```python
from build123d import *

# Parameters (mm, degrees)
BOSS_EXTRU_3_DEPTH      = 30
ESQUISSE2_W             = 15
ESQUISSE2_H             = 50
BOSS_EXTRU_4_DEPTH      = 30
CONG_1_R                = 5
ESQUISSE3_R             = 4
ENL_V_MAT_EXTRU_1_DEPTH = 30
ESQUISSE4_R             = 4
ENL_V_MAT_EXTRU_2_DEPTH = 30
CONG_2_R                = 0.5
ESQUISSE5_R             = 3
ENL_V_MAT_EXTRU_3_DEPTH = 30


with BuildPart() as part:
    # Esquisse1 → Boss.-Extru.3 (new body)
    with BuildSketch(Plane.XY):
        with BuildLine():
            Line((-1.516636282, -1.472839764), (-164.999487802, -160.23473102))
            ThreePointArc((-164.999487802, -160.23473102), (-168.55609482, -161.647249147), (-172.069796906, -160.131149351))
            Line((-172.069796906, -160.131149351), (-182.523190666, -149.366912378))
            ThreePointArc((-182.523190666, -149.366912378), (-186.036892752, -147.850812582), (-189.593499771, -149.263330708))
            Line((-189.593499771, -149.263330708), (-193.180445158, -152.746694426))
            ThreePointArc((-193.180445158, -152.746694426), (-194.696544953, -156.260396513), (-193.284026827, -159.817003531))
            Line((-193.284026827, -159.817003531), (-179.34726935, -174.168185892))
            Line((-179.34726935, -174.168185892), (-168.352304295, -185.490098382))
            ThreePointArc((-168.352304295, -185.490098382), (-164.775881538, -187.006723591), (-161.193106921, -185.505165132))
            Line((-161.193106921, -185.505165132), (-37.640520995, -59.345455931))
            ThreePointArc((-37.640520995, -59.345455931), (-34.371026094, -57.123623648), (-30.496017021, -56.342316868))
            Line((-30.496017021, -56.342316868), (10, -56.342316868))
            ThreePointArc((10, -56.342316868), (13.535533906, -54.877850774), (15, -51.342316868))
            Line((15, -51.342316868), (15, -6.342316868))
            Line((15, -6.342316868), (15, 50))
            Line((15, 50), (5, 50))
            ThreePointArc((5, 50), (1.464466094, 48.535533906), (0, 45))
            Line((0, 45), (0, 2.114105623))
            ThreePointArc((0, 2.114105623), (-0.394741126, 0.166904887), (-1.516636282, -1.472839764))
        make_face()
    extrude(amount=BOSS_EXTRU_3_DEPTH)

    # Esquisse2 → Boss.-Extru.4 (add)
    with BuildSketch(Plane.XY):
        with Locations((7.5, -76.342316868)):
            Rectangle(ESQUISSE2_W, ESQUISSE2_H)
    extrude(amount=BOSS_EXTRU_4_DEPTH)

    # Congé1
    cong_1_edges = [part.edges().sort_by_distance(p)[0] for p in [
        (0, -56.342316868, 15),
        (0, -101.342316868, 15),
    ]]
    fillet(cong_1_edges, radius=CONG_1_R)

    # Esquisse3 → Enlèv. mat.-Extru.1 (cut)
    with BuildSketch(Plane.ZY):
        with Locations((15, 23.557052811)):
            Circle(ESQUISSE3_R)
    extrude(amount=-ENL_V_MAT_EXTRU_1_DEPTH, mode=Mode.SUBTRACT)

    # Esquisse4 → Enlèv. mat.-Extru.2 (cut)
    with BuildSketch(Plane.ZY):
        with Locations((15, -78.842316868)):
            Circle(ESQUISSE4_R)
    extrude(amount=-ENL_V_MAT_EXTRU_2_DEPTH, mode=Mode.SUBTRACT)

    # Congé2
    cong_2_edges = [part.edges().sort_by_distance(p)[0] for p in [
        (0, 23.557052811, 11),
        (0, -78.842316868, 11),
    ]]
    fillet(cong_2_edges, radius=CONG_2_R)

    # Esquisse5 → Enlèv. mat.-Extru.3 (cut)
    with BuildSketch(Plane.XY.offset(30)):
        with Locations((-7.637173742, -35.95688684)):
            Circle(ESQUISSE5_R)
    extrude(amount=-ENL_V_MAT_EXTRU_3_DEPTH, mode=Mode.SUBTRACT)


solid = part.part
```
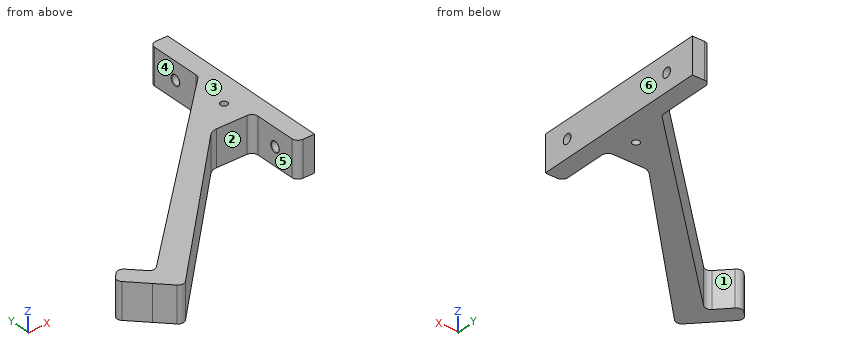
Read the model definition and answer for the solid it produces. Units are mm, in the model's axes. Face numbers are marked on the shaded views. A direction names the side the tool comes from. Round coordinates to 2 decimals unless told otherwise and drop trailing zeros. Loops run counter-clockwise (first coordinate to the right, second up) from the corner with the lowest first, then second, coordinate; pieces in that order, holes last. Notation, with made-up numbers: (69.25, 55.25) -> (88.25, 55.25) arc R24 ccw to (88.25, 70.25) -> close; hole circle Ø2 at (84, 34.25). An arc over 180 degrees is marked (long way). One line per item, written item: value.
1) A cutting plane is placed at C-C (y = -107.5). Determine the outline of the cut face in (x, z), and give its area (3 significant figures).
Answer list:
outline: (-110.7, 0) -> (-84.8, 0) -> (-84.8, 30) -> (-110.7, 30) -> close
area: 777 mm²
2) Consider L1, parallel to Y at x = 6.5, z = 15; L2, parallel to Y at x = 4, z = 15; L3, parallel to X at y = -85, z = 15.5. Determine where each line is inside the solid, lowest interval first. Write a range as [from, to].
Answer list:
L1: y = [-101.34, -82.84], [-74.84, 19.56], [27.56, 50]
L2: y = [-101.24, -82.84], [-74.84, 19.56], [27.56, 49.9]
L3: x = [-87.53, -62.76], [0, 15]
3) For the marked faces 1, 2 and 3, determine the directions among +Z, -Z, +X, -X, +Y, -Y from which every point of the face is accessible in a straight line to the end or side of a thin tool.
Answer list:
face 1: +Z, -Z, +Y
face 2: +Z, -Z, -Y
face 3: +Z, +X, -X, +Y, -Y
4) Flat-ended cylindrical pins translate along their axes: P1, Ø10, axis at x = -72, z = 24, coming from the -Y side; P2, Ø3, axis at x = -55.5, z = 21.5, coming from the +Y side; P3, Ø8, axis at y = -138, z = 25, coming from the -X side; P4, Ø7, axis at y = 23.56, z = 15, coming from the +X side. Find the tip coordinate at first contact, or state that the pin passes through.
Answer list:
P1: stops at y = -99.54
P2: stops at y = -52.44
P3: stops at x = -146.22
P4: passes through
5) A cutting plane is placed at D-D (x = -20.5). Determine the outline of the cut face in (y, z), and give its area (3 significant figures).
Answer list:
outline: (-56.34, 0) -> (-19.91, 0) -> (-19.91, 30) -> (-56.34, 30) -> close
area: 1,090 mm²
6) The mould has two halves that part along X. Classify the marked faces 4, 5 and 6: pulls with the +X half, pulls with the -X half, needs draft (parallel to the pull), parting line crosses it, or undercut.
Answer list:
face 4: pulls with the -X half
face 5: undercut
face 6: pulls with the +X half
7) A cutting plane is placed at B-B (z = 3). Determine the outline of the cut face in (x, y).
Answer list:
outline: (-193.28, -159.82) -> (-168.35, -185.49) arc R5 ccw to (-161.19, -185.51) -> (-37.64, -59.35) arc R10 cw to (-30.5, -56.34) -> (-5, -56.34) arc R5 cw to (0, -61.34) -> (0, -96.34) arc R5 ccw to (5, -101.34) -> (15, -101.34) -> (15, 50) -> (5, 50) arc R5 ccw to (0, 45) -> (0, 2.11) arc R5 cw to (-1.52, -1.47) -> (-165, -160.23) arc R5 cw to (-172.07, -160.13) -> (-182.52, -149.37) arc R5 ccw to (-189.59, -149.26) -> (-193.18, -152.75) arc R5 ccw to start; hole circle Ø6 at (-7.64, -35.96)
8) A cutting plane is placed at A-A (z = 15). Give the number of separate pieces and of enclosed holes in the cut face, and give its area (3 significant figures).
Answer list:
separate pieces: 3
enclosed holes: 1
area: 7,310 mm²
